The figure shows three views and two pictorial views of one solid part (mm, origin at its lowest corner). Answer the questions. Coordinates: 2 decimals unless noted, no trailing zeros. Write each loop counter-clockwise with the first axis right and the second up, starting at its lowest first coordinate (ties: lowest second). Pieces come first, ordered by that corner, then holes.
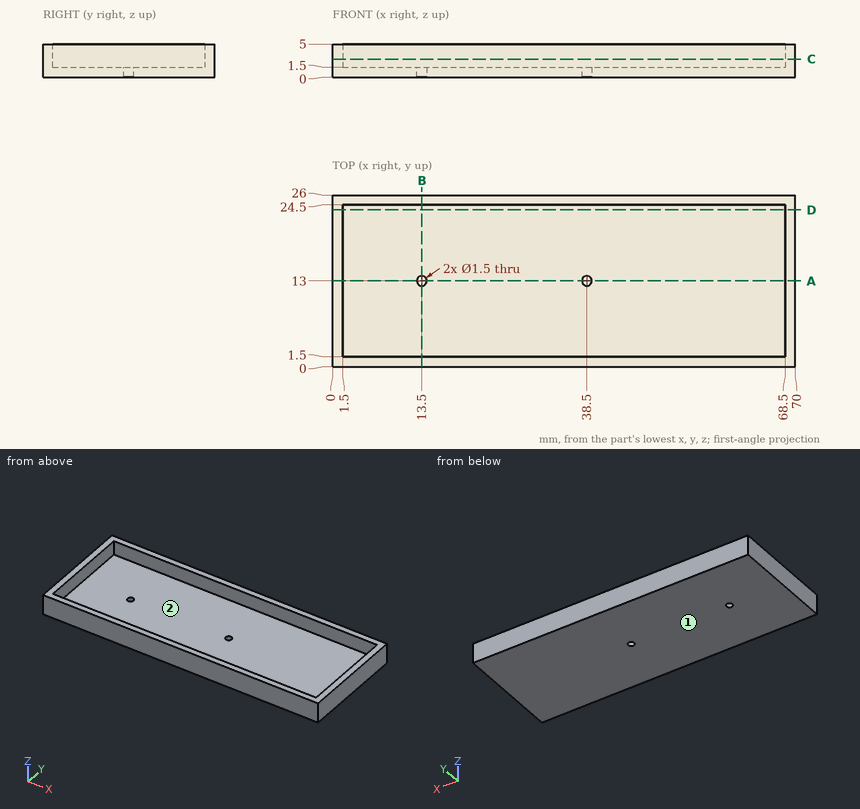
1. A flat-ended cylindrical pin translates along its axis: P1, Ø2, axis at x = 13.5, y = 13, coming from the +Z side. Find the tip coordinate at first contact, or state that the pin passes through.
Results found:
P1: stops at z = 1.5
2. Section A-A on y = 13 is taken. Give the vertices of the cut face in (x, z).
Results found:
outline: (0, 0) - (12.75, 0) - (12.75, 1.5) - (1.5, 1.5) - (1.5, 5) - (0, 5) - close; (14.25, 0) - (37.75, 0) - (37.75, 1.5) - (14.25, 1.5) - close; (39.25, 0) - (70, 0) - (70, 5) - (68.5, 5) - (68.5, 1.5) - (39.25, 1.5) - close
3. Find the intervals of material crossed by L1, parallel to Y at x = 13.5, z = 0.5; L2, parallel to Y at x = 44.5, z = 1.75; L3, parallel to X at y = 7.25, z = 2.2, in increasing order.
Results found:
L1: y = 0 to 12.25, 13.75 to 26
L2: y = 0 to 1.5, 24.5 to 26
L3: x = 0 to 1.5, 68.5 to 70
4. Section B-B on x = 13.5 is taken. Give the vertices of the cut face in (y, z).
Results found:
outline: (0, 0) - (12.25, 0) - (12.25, 1.5) - (1.5, 1.5) - (1.5, 5) - (0, 5) - close; (13.75, 0) - (26, 0) - (26, 5) - (24.5, 5) - (24.5, 1.5) - (13.75, 1.5) - close
5. For a pull along X with two mould halves and no side action, classify the marked faces 1 and 2 as pulls with the +X half, pulls with the -X half, needs draft (parallel to the pull), parting line crosses it, or undercut.
Results found:
face 1: needs draft
face 2: undercut
6. Section C-C on z = 2.7 is taken. Give the vertices of the cut face in (x, y), then the cut area to 3 significant figures.
Results found:
outline: (0, 0) - (70, 0) - (70, 26) - (0, 26) - close; hole (1.5, 1.5) - (68.5, 1.5) - (68.5, 24.5) - (1.5, 24.5) - close
area: 279 mm2
7. Section D-D on y = 23.75 is taken. Give the vertices of the cut face in (x, z), then the cut area to 4 significant figures.
Results found:
outline: (0, 0) - (70, 0) - (70, 5) - (68.5, 5) - (68.5, 1.5) - (1.5, 1.5) - (1.5, 5) - (0, 5) - close
area: 115.5 mm2
